Input: part model. Units: mm. Frame: model coordinates. A direction names the side the tool comes from. Round coordinates to 2 decimals unless told otherwise and drop trailing zeros. Order: outer loops, then holes, each group sorted by start corner. A loop starts at its lowest first (then second) coordinate and runs counter-clockwise, first axis right, second up. Notation, with made-up numbers: M 27.5,20 L 81.5,20 A23 ccw 81.5,52 Z; hole C -39,52.25 d9. An arc over 180 degrees is marked long. One line per question, with ' | ' between items.
```python
from build123d import *

# Parameters (mm, degrees)
SKETCH1_R                = 1
BOSS_EXTRUDE1_DEPTH      = 1.15
SKETCH2_W                = 22.7
SKETCH2_H                = 10.1
BOSS_EXTRUDE2_DEPTH      = 5.9
BOSS_EXTRUDE3_DEPTH      = 2
BOSS_EXTRUDE3_DEPTH_BACK = 0.5
SKETCH3_R                = 0.68


with BuildPart() as part:
    # Sketch1 → Boss-Extrude1 (new body)
    with BuildSketch(Plane(origin=(0, 0, 0), x_dir=(1, 0, 0), z_dir=(0, 1, 0))):
        Polygon((-12.5, 6.5), (12.5, 6.5), (12.5, 2.5), (14.9, 2.5), (14.9, -2.5), (12.5, -2.5), (12.5, -6.5), (-12.5, -6.5), (-12.5, -2.5), (-14.9, -2.5), (-14.9, 2.5), (-12.5, 2.5), align=None)
        with Locations(Location((13.06, 0, 0), (0, 0, 270))):
            Circle(SKETCH1_R, mode=Mode.SUBTRACT)
        with Locations(Location((-13.06, 0, 0), (0, 0, 270))):
            Circle(SKETCH1_R, mode=Mode.SUBTRACT)
    extrude(amount=BOSS_EXTRUDE1_DEPTH)

    # Sketch2 → Boss-Extrude2 (add)
    with BuildSketch(Plane(origin=(0, 1.15, 0), x_dir=(1, 0, 0), z_dir=(0, 1, 0))):
        Rectangle(SKETCH2_W, SKETCH2_H)
    extrude(amount=BOSS_EXTRUDE2_DEPTH)

    # Sketch3 → Boss-Extrude3 (add, two sides: drawn at the far end of the back side and taken through both)
    with BuildSketch(Plane(origin=(0, 0, -6.5), x_dir=(-1, 0, 0), z_dir=(0, 0, -1)).offset(-BOSS_EXTRUDE3_DEPTH_BACK)):
        with Locations((8.85, 0)):
            Circle(SKETCH3_R)
        with Locations((6.35, 0)):
            Circle(SKETCH3_R)
    extrude(amount=BOSS_EXTRUDE3_DEPTH + BOSS_EXTRUDE3_DEPTH_BACK)


solid = part.part
```
Item 1: Section query C-C, the plane z = -1.5. Return loops of the section in (x, y), plus the area to 3 significant figures.
Report:
outline: M -14.9,0 L 14.9,0 L 14.9,1.15 L 11.35,1.15 L 11.35,7.05 L -11.35,7.05 L -11.35,1.15 L -14.9,1.15 Z | area: 168 mm²
Item 2: Line query: line 1 along X through (y, z) = (0.45, 0); line 2 along Y through (x, z) = (11, -2.75); line 3 along Z through (x, y) = (11.25, 0.25). Output: solid intervals per line, ascending. Write a range as from..to.
Report:
line 1: -14.9..-14.06, -12.06..12.06, 14.06..14.9 | line 2: 0..7.05 | line 3: -6.5..6.5
Item 3: Access query for faces 1 (the flat face through (-13.7, 0.6, 2.5)), 2 (the flat face through (0, 4, -5.05)), 3 (the flat face through (11.35, 4, 0)), 4 (the flat face through (-13.7, 0.6, -2.5)). Directions: +Z, -Z, +X, -X, +Y, -Y. A direction counts if a zero-diameter tool reaches every point of the face in a straight line with its end or side. Return the directions, or none.
Report:
face 1: +Z, -X, +Y, -Y | face 2: -Z, +X, -X, +Y | face 3: +Z, -Z, +X, +Y | face 4: -Z, -X, +Y, -Y
Item 4: Section query D-D, the plane y = 6.25. Return loops of the section in (x, z).
Report:
outline: M -11.35,-5.05 L 11.35,-5.05 L 11.35,5.05 L -11.35,5.05 Z
Item 5: Mould query, pull axis X, two halves, no side actions, for faces 5 (the flat face through (12.5, 0.6, 4.5)), 6 (the flat face through (-11.35, 4, 0)), 7 (the flat face through (-6, 0, -8.5)), 8 (the cylindrical face through (-6.664, -0.603, -7.232)). Classes: +X half, -X half, draft (parallel to the pull), parting line (faces both ways), or undercut.
Report:
face 5: +X half | face 6: -X half | face 7: draft | face 8: undercut
Item 6: Section query A-A, the plane x = 13.06. Return loops of the section in (y, z).
Report:
outline: M 0,-2.5 L 1.15,-2.5 L 1.15,-1 L 0,-1 Z; M 0,1 L 1.15,1 L 1.15,2.5 L 0,2.5 Z
Item 7: First-contact query: pin 1 (1.2 mm diameter, centred on x = -13.06, z = 0, fed in from -Y); pin 2 (0.6 mm diameter, centred on x = 14.5, y = 0.5, fed in from +Z); pin 3 (2.5 mm diameter, centred on x = 13.06, z = 0, fed in from +Y); pin 4 (1.3 mm diameter, centred on x = -13, y = 0.5, fed in from -Z). Flat tips, straight axial feed; report the tip coordinate or a pass-through.
Report:
pin 1: through | pin 2: z = 2.5 | pin 3: y = 1.15 | pin 4: z = -6.5
Item 8: Section query B-B, the plane x = -1.75. Return loops of the section in (y, z), plus the area to 3 significant figures.
Report:
outline: M 0,-6.5 L 1.15,-6.5 L 1.15,-5.05 L 7.05,-5.05 L 7.05,5.05 L 1.15,5.05 L 1.15,6.5 L 0,6.5 Z | area: 74.5 mm²
